Geometry: final body of the model. Coordinates: model frame, mm. Give positions to 0.01 mm unless a question says otherwise; leave off trailing zeros. Write each loop counter-clockwise with the first axis right and the second up, starting at its lowest first coordinate (ties: lowest second). Pieces come first, ordered by that corner, then holes. Notation, with made-up numbers: M 25,37 L 64,37 A26 ccw 64,61 Z; hole C 31,55.5 d3. An arc over 180 degrees is marked long. Use a Markdown table: item, result. Add a question column.
1) Section B-B on z = 2.85. Return the cut outline in (x, y) (1 decimal), then the cut area to 3 significant figures.
2) Section A-A on x = 2.5. Return the cut outline in (y, z) (1 decimal).
3) Draft query along Y for faces 1 (the flat face through (2, 16.245, 2)), 2 (the flat face through (0, 8, 2)), 3 (the cylindrical face through (2.98, 3.37, 2.06)), 4 (the flat face through (2, 0, 2)). Return one class per face: +Y half, -Y half, draft (parallel to the pull), parting line (faces both ways), or undercut.
4) Line query: line 1 (Y direction, x = 2.5, z = 1.95) (1 decimal); line 2 (Y direction, x = 1.75, z = 0.35) (3 decimals); line 3 (X direction, y = 3, z = 1.1). Output: solid intervals per line, ascending.
```python
from build123d import *

# Parameters (mm, degrees)
ESBO_O1_W                = 5
ESBO_O1_H                = 16.245
ESBO_O1_R                = 0.889
RESSALTO_EXTRUS_O1_DEPTH = 4.064


with BuildPart() as part:
    # Esboço1 → Ressalto-extrusão1 (new body)
    with BuildSketch(Plane.XY.offset(4.064)):
        with Locations((2.5, 8.1225)):
            Rectangle(ESBO_O1_W, ESBO_O1_H)
        with Locations((2.5, 2.6225)):
            Circle(ESBO_O1_R, mode=Mode.SUBTRACT)
        with Locations((2.5, 13.6225)):
            Circle(ESBO_O1_R, mode=Mode.SUBTRACT)
    extrude(amount=-RESSALTO_EXTRUS_O1_DEPTH)


solid = part.part
```
Found:
| question | item | result |
|---|---|---|
| 1 | outline | M 0,0 L 5,0 L 5,16.2 L 0,16.2 Z; hole C 2.5,2.6 d1.8; hole C 2.5,13.6 d1.8 |
| 1 | area | 76.3 mm² |
| 2 | outline | M 0,0 L 1.7,0 L 1.7,4.1 L 0,4.1 Z; M 3.5,0 L 12.7,0 L 12.7,4.1 L 3.5,4.1 Z; M 14.5,0 L 16.2,0 L 16.2,4.1 L 14.5,4.1 Z |
| 3 | face 1 | +Y half |
| 3 | face 2 | draft |
| 3 | face 3 | undercut |
| 3 | face 4 | -Y half |
| 4 | line 1 | 0 to 1.7, 3.5 to 12.7, 14.5 to 16.2 |
| 4 | line 2 | 0 to 2.145, 3.1 to 13.145, 14.1 to 16.245 |
| 4 | line 3 | 0 to 1.7, 3.3 to 5 |
